The listing builds one solid part. Answer for the finished solid, in the listing's coordinates (mm). A direction names the side the tool comes from. Coordinates: 2 decimals unless noted, no trailing zeros. Return JSON: item names as keys, results as strings.
```python
from build123d import *

# Parameters (mm, degrees)
SKETCH1_R                = 60
SKETCH1_R_2              = 12.5
BOSS_EXTRUDE1_DEPTH      = 12.5
SKETCH2_R                = 42.5
CUT_EXTRUDE1_DEPTH       = 10
SKETCH3_R                = 6
CUT_EXTRUDE2_DEPTH       = 16
CIRPATTERN1_COUNT        = 5
SKETCH5_R                = 13.5
SKETCH5_R_2              = 12.5
BOSS_EXTRUDE2_DEPTH      = 2
BOSS_EXTRUDE2_DEPTH_BACK = 7


with BuildPart() as part:
    # Sketch1 → Boss-Extrude1 (new body, symmetric)
    with BuildSketch(Plane.XY):
        Circle(SKETCH1_R)
        Circle(SKETCH1_R_2, mode=Mode.SUBTRACT)
    extrude(amount=BOSS_EXTRUDE1_DEPTH, both=True)

    # Sketch2 → Cut-Extrude1 (cut)
    with BuildSketch(Plane.XY.offset(12.5)):
        Circle(SKETCH2_R)
    cut_extrude1 = extrude(amount=-CUT_EXTRUDE1_DEPTH, mode=Mode.SUBTRACT)

    # Mirror1: Cut-Extrude1 across plane
    add(cut_extrude1.mirror(Plane.XY), mode=Mode.SUBTRACT)

    # Sketch3 → Cut-Extrude2 (cut, through all)
    with BuildSketch(Plane.XY.offset(2.5)):
        with Locations((0, 25)):
            Circle(SKETCH3_R)
    cut_extrude2 = extrude(amount=-CUT_EXTRUDE2_DEPTH, mode=Mode.SUBTRACT)

    # CirPattern1: Cut-Extrude2 ×5 about axis
    cirpattern1_axis = Axis((0, 0, 0), (0, 0, 1))
    for i in range(1, CIRPATTERN1_COUNT):
        add(cut_extrude2.rotate(cirpattern1_axis, i * 360 / CIRPATTERN1_COUNT), mode=Mode.SUBTRACT)

    # Sketch4 → Cut-Revolve1 (revolve, cut)
    with BuildSketch(Plane(origin=(0, 0, 0), x_dir=(1, 0, 0), z_dir=(0, 1, 0))):
        Polygon((60, 9.5), (54, 6.035898385), (54, -6.035898385), (60, -9.5), align=None)
    revolve(axis=Axis((0, 0, 0), (0, 0, -1)), mode=Mode.SUBTRACT)

    # Sketch5 → Boss-Extrude2 (add, two sides)
    with BuildSketch(Plane.XY.offset(2.5)) as boss_extrude2_sk:
        Circle(SKETCH5_R)
        Circle(SKETCH5_R_2, mode=Mode.SUBTRACT)
    extrude(amount=BOSS_EXTRUDE2_DEPTH)
    extrude(boss_extrude2_sk.sketch, amount=-BOSS_EXTRUDE2_DEPTH_BACK)


solid = part.part
```
Item 1: Determine the mould class of faces 1 (the flat face through (12, 41, -12.5)), 2 (the conical face through (-11.79, 53.08, 6.25)), 3 (the cylindrical face through (-2.93, -13.18, -3.49)) for opening direction X: pulls with the +X half, pulls with the -X half, needs draft (parallel to the pull), parting line crosses it, or undercut.
Answer list:
{"face 1": "needs draft", "face 2": "parting line crosses it", "face 3": "undercut"}
Item 2: Which of the six approach directions +Z, -Z, +X, -X, +Y, -Y give full straight-line access (tool end or side, diameter ignored) to faces 4 (the cylindrical face through (-59.94, 2.64, -10.98)), 5 (the flat face through (9, -9, 4.5)), 6 (the cylindrical face through (-33.727, -25.861, -7.57)), 7 (the cylindrical face through (-11.706, 52.716, 0.085))?
Answer list:
{"face 4": "+Z, -Z", "face 5": "+Z", "face 6": "-Z", "face 7": "none"}
Item 3: The part is cut by section B-B on x = 0. Count the separate pieces of the cut face and the enclosed holes in it, plus the area to 3 significant figures.
Answer list:
{"separate pieces": "3", "enclosed holes": "0", "area": "937 mm2"}
Item 4: Flat-ended cylindrical pins translate along their axes: pin 1 (14 mm diameter, centred on x = 23.78, y = 7.73, fed in from -Z); pin 2 (3 mm diameter, centred on y = 30.5, z = -7, fed in from -X); pin 3 (5 mm diameter, centred on x = 33, z = 2, fed in from +Y). Find the tip coordinate at first contact, or state that the pin passes through.
Answer list:
{"pin 1": "z = -2.5", "pin 2": "x = -49.78", "pin 3": "y = 44.56"}
Item 5: Find the intervals of material crossed by probe 1 along Y at (x, z) = (0, 0.7); probe 2 along Y at (x, z) = (0, -3.85); probe 3 along X at (y, z) = (1.5, 3.75), in increasing order.
Answer list:
{"probe 1": "-54 to -12.5, 12.5 to 19, 31 to 54", "probe 2": "-54 to -42.5, -13.5 to -12.5, 12.5 to 13.5, 42.5 to 54", "probe 3": "-53.98 to -42.47, -13.42 to -12.41, 12.41 to 13.42, 42.47 to 53.98"}
